```python
from build123d import *

# Parameters (mm, degrees)
F1_DEPTH = 16.2814
F2_R     = 0.254
F4_DEPTH = 25.4
F6_DEPTH = 79.9094


with BuildPart() as f1:
    # F0 (on Front) → F1 (new body)
    with BuildSketch(Plane.XZ):
        with BuildLine():
            Line((75.5142, 0), (79.9084, 0))
            ThreePointArc((79.9084, 0), (39.9542, 39.9542), (0, 0))
            Line((0, 0), (4.3942, 0))
            ThreePointArc((4.3942, 0), (39.9542, 35.56), (75.5142, 0))
        make_face()
    extrude(amount=F1_DEPTH)

    # F2
    f2_edges = [f1.edges().sort_by_distance(p)[0] for p in [
        (39.9542, -16.2814, 39.9542),
        (39.9542, -16.2814, 35.56),
        (39.9542, 0, 39.9542),
        (39.9542, 0, 35.56),
    ]]
    fillet(f2_edges, radius=F2_R)

    # F3 (on face) → F4 (join)
    with BuildSketch(Plane(origin=(0, 0, 0), x_dir=(1, 0, 0), z_dir=(0, 0, -1))):
        with BuildLine():
            ThreePointArc((0.254, 16.2814), (0.074395, 16.207005), (0, 16.0274))
            Line((0, 16.0274), (0, 0.254))
            ThreePointArc((0, 0.254), (0.074395, 0.074395), (0.254, 0))
            Line((0.254, 0), (4.1402, 0))
            ThreePointArc((4.1402, 0), (4.319805, 0.074395), (4.3942, 0.254))
            Line((4.3942, 0.254), (4.3942, 16.0274))
            ThreePointArc((4.3942, 16.0274), (4.319805, 16.207005), (4.1402, 16.2814))
            Line((4.1402, 16.2814), (0.254, 16.2814))
        make_face()
        with BuildLine():
            ThreePointArc((75.5142, 0.254), (75.588595, 0.074395), (75.7682, 0))
            Line((75.7682, 0), (79.6544, 0))
            ThreePointArc((79.6544, 0), (79.834005, 0.074395), (79.9084, 0.254))
            Line((79.9084, 0.254), (79.9084, 16.0274))
            ThreePointArc((79.9084, 16.0274), (79.834005, 16.207005), (79.6544, 16.2814))
            Line((79.6544, 16.2814), (75.7682, 16.2814))
            ThreePointArc((75.7682, 16.2814), (75.588595, 16.207005), (75.5142, 16.0274))
            Line((75.5142, 16.0274), (75.5142, 0.254))
        make_face()
    extrude(amount=F4_DEPTH)

    # F5 (on face) → F6 (cut, through all)
    with BuildSketch(Plane(origin=(0, 0, 0), x_dir=(0, -1, 0), z_dir=(-1, 0, 0))):
        with BuildLine():
            ThreePointArc((16.2814, -17.2593), (8.1407, -25.4), (0, -17.2593))
            Line((0, -17.2593), (0, -26.5704))
            Line((0, -26.5704), (16.2814, -26.5704))
            Line((16.2814, -26.5704), (16.2814, -17.2593))
        make_face()
    extrude(amount=-F6_DEPTH, mode=Mode.SUBTRACT)


solid = f1.part
```
Here's how the part is built. I have some questions about the finished solid (model axes, mm). A direction names the side the tool comes from. Coordinates: 2 decimals unless noted, no trailing zeros. Loops run counter-clockwise (first coordinate to the right, second up) from the corner with the lowest first, then second, coordinate; pieces in that order, holes last. Notation, with made-up numbers: (8, 41.5) -> (65, 41.5) arc R32 cw to (65, 67.5) -> close; hole circle Ø3 at (-0.75, 5.25). An arc over 180 degrees is marked (long way). Return JSON: item names as keys, results as strings.
1) Thinking about a two-plate mould opening in X: for faces 3 (the face through (40, -16.281, 37)), 4 (the face through (39.17, -8.03, 35.55)), 5 (the face through (40.833, -8.03, 39.945)), 6 (the face through (0, -8, -13)), which applies, +X half, -X half, draft (parallel to the pull), parting line (faces both ways), or undercut?
Results below:
{"face 3": "draft", "face 4": "undercut", "face 5": "parting line", "face 6": "-X half"}
2) For faces 1 (the face through (2.2, -8.3, -25.4)), 2 (the face through (75.514, -8, -13)), which set-ups out of +Z, -Z, +X, -X, +Y, -Y let a thin tool reach every point of the face, with its end or its side?
Results below:
{"face 1": "-Z, +X, -X", "face 2": "-Z, +Y, -Y"}
3) If we section it at C-C, the plane y = -5: Write out the boundary of the cut face in (x, z), then the cut area to 3 significant figures.
Results below:
{"outline": "(0, -24.77) -> (4.39, -24.77) -> (4.39, 0) arc R35.56 cw to (75.51, 0) -> (75.51, -24.77) -> (79.91, -24.77) -> (79.91, 0) arc R39.95 ccw to (0, 0) -> close", "area": "739 mm²"}
4) If we section it at B-B, the plane y = -12: Write out the boundary of the cut face in (x, z).
Results below:
{"outline": "(0, -24.43) -> (4.39, -24.43) -> (4.39, 0) arc R35.56 cw to (75.51, 0) -> (75.51, -24.43) -> (79.91, -24.43) -> (79.91, 0) arc R39.95 ccw to (0, 0) -> close"}
5) Will these pins go through, and if not, where does the flat tip stop? pin 1 (5 mm diameter, centred on x = 45.5, y = -8.5, fed in from +Z); pin 2 (4 mm diameter, centred on y = -5, z = 32.5, fed in from +X).
Results below:
{"pin 1": "z = 39.84", "pin 2": "x = 65.76"}
6) I need wall thicknesses on line 1 (X direction, y = -11.5, z = 0); line 2 (X direction, y = -6, z = 25); line 3 (Z direction, x = 41, y = -4.25). Which ranges of each line are inside material? Lowest first, please. Write a range as from..to.
Results below:
{"line 1": "0..4.39, 75.51..79.91", "line 2": "8.79..14.67, 65.24..71.12", "line 3": "35.54..39.94"}
7) If we section it at A-A, the plane z = -5.5: Write out the boundary of the cut face in (x, y).
Results below:
{"outline": "(0, -16.03) arc R0.25 ccw to (0.25, -16.28) -> (4.14, -16.28) arc R0.25 ccw to (4.39, -16.03) -> (4.39, -0.25) arc R0.25 ccw to (4.14, 0) -> (0.25, 0) arc R0.25 ccw to (0, -0.25) -> close; (75.51, -16.03) arc R0.25 ccw to (75.77, -16.28) -> (79.65, -16.28) arc R0.25 ccw to (79.91, -16.03) -> (79.91, -0.25) arc R0.25 ccw to (79.65, 0) -> (75.77, 0) arc R0.25 ccw to (75.51, -0.25) -> close"}
